CAD build for the part. Positions are in the model's coordinates, mm. A direction names the side the tool comes from. Coordinates: 2 decimals unless noted, no trailing zeros. Loops run counter-clockwise (first coordinate to the right, second up) from the corner with the lowest first, then second, coordinate; pieces in that order, holes last. Notation, with made-up numbers: (61, -19) -> (110, -19) arc R17 cw to (110, 11) -> close; hole circle Ø2 at (16, 66). An arc over 180 degrees is marked (long way). Write each question's results on one line, items separated by ' | '.
from build123d import *

# Parameters (mm, degrees)
SKETCH1_R           = 7
SKETCH1_R_2         = 1.75
BOSS_EXTRUDE1_DEPTH = 3
SKETCH2_R           = 4
SKETCH2_R_2         = 1.75
BOSS_EXTRUDE2_DEPTH = 6
FILLET1_R           = 3
SKETCH4_R           = 2.75
SKETCH4_R_2         = 1.75
BOSS_EXTRUDE3_DEPTH = 4.25


# Some blends are built 0.0001 mm under size
with BuildPart() as part:
    # Sketch1 → Boss-Extrude1 (new body)
    with BuildSketch(Plane(origin=(0, 0, 0), x_dir=(0, 0, -1), z_dir=(1, 0, 0))):
        Circle(SKETCH1_R)
        Circle(SKETCH1_R_2, mode=Mode.SUBTRACT)
    extrude(amount=BOSS_EXTRUDE1_DEPTH)

    # Sketch2 → Boss-Extrude2 (add)
    with BuildSketch(Plane(origin=(3, 0, 0), x_dir=(0, 0, -1), z_dir=(1, 0, 0))):
        Circle(SKETCH2_R)
        Circle(SKETCH2_R_2, mode=Mode.SUBTRACT)
    extrude(amount=BOSS_EXTRUDE2_DEPTH)

    # Fillet1
    fillet1_edges = [part.edges().sort_by_distance(p)[0] for p in [
        (3, 0, 4),
    ]]
    fillet(fillet1_edges, radius=FILLET1_R - 0.0001)  # a hair under: the kernel refuses the full size

    # Sketch4 → Boss-Extrude3 (add)
    with BuildSketch(Plane(origin=(9, 0, 0), x_dir=(0, 0, -1), z_dir=(1, 0, 0))):
        Circle(SKETCH4_R)
        Circle(SKETCH4_R_2, mode=Mode.SUBTRACT)
    extrude(amount=BOSS_EXTRUDE3_DEPTH)

    # Chamfer1
    # the kernel refuses this chamfer: 0.25 mm, written as the material it takes off along each edge
    with BuildSketch(Plane(origin=(9, 0, 0), x_dir=(0, 0, -1), z_dir=(0, -1, 0))) as chamfer1_piece_1:
        with BuildLine():
            Line((3.696966991, 0.053033009), (4.053033009, -0.303033009))
            Line((4.053033009, -0.303033009), (4.090533009, -0.303033009))
            ThreePointArc((4.090533009, -0.303033009), (4.0375, -0.151516504), (4.0375, 0))
            Line((4.0375, 0), (4, 0.0375))
            ThreePointArc((4, 0.0375), (3.848483496, 0.0375), (3.696966991, 0.090533009))
            Line((3.696966991, 0.090533009), (3.696966991, 0.053033009))
        make_face()
    revolve(axis=Axis((9, 0, 0), (1, 0, 0)), mode=Mode.SUBTRACT)
    with BuildSketch(Plane(origin=(0, 0, 0), x_dir=(0, 0, -1), z_dir=(0, -1, 0))) as chamfer1_piece_2:
        with BuildLine():
            Line((7.053033009, 0.303033009), (6.696966991, -0.053033009))
            Line((6.696966991, -0.053033009), (6.696966991, -0.090533009))
            ThreePointArc((6.696966991, -0.090533009), (6.848483496, -0.0375), (7, -0.0375))
            Line((7, -0.0375), (7.0375, 0))
            ThreePointArc((7.0375, 0), (7.0375, 0.151516504), (7.090533009, 0.303033009))
            Line((7.090533009, 0.303033009), (7.053033009, 0.303033009))
        make_face()
    revolve(axis=Axis((0, 0, 0), (1, 0, 0)), mode=Mode.SUBTRACT)
    with BuildSketch(Plane(origin=(13.25, 0, 0), x_dir=(0, 0, -1), z_dir=(0, -1, 0))) as chamfer1_piece_3:
        with BuildLine():
            Line((2.446966991, 0.053033009), (2.803033009, -0.303033009))
            Line((2.803033009, -0.303033009), (2.840533009, -0.303033009))
            ThreePointArc((2.840533009, -0.303033009), (2.7875, -0.151516504), (2.7875, 0))
            Line((2.7875, 0), (2.75, 0.0375))
            ThreePointArc((2.75, 0.0375), (2.598483496, 0.0375), (2.446966991, 0.090533009))
            Line((2.446966991, 0.090533009), (2.446966991, 0.053033009))
        make_face()
    revolve(axis=Axis((13.25, 0, 0), (1, 0, 0)), mode=Mode.SUBTRACT)
    with BuildSketch(Plane(origin=(3, 0, 0), x_dir=(0, 0, -1), z_dir=(0, -1, 0))) as chamfer1_piece_4:
        with BuildLine():
            Line((6.696966991, 0.053033009), (7.053033009, -0.303033009))
            Line((7.053033009, -0.303033009), (7.090533009, -0.303033009))
            ThreePointArc((7.090533009, -0.303033009), (7.0375, -0.151516504), (7.0375, 0))
            Line((7.0375, 0), (7, 0.0375))
            ThreePointArc((7, 0.0375), (6.848483496, 0.0375), (6.696966991, 0.090533009))
            Line((6.696966991, 0.090533009), (6.696966991, 0.053033009))
        make_face()
    revolve(axis=Axis((3, 0, 0), (1, 0, 0)), mode=Mode.SUBTRACT)
    with BuildSketch(Plane(origin=(0, 0, 0), x_dir=(0, 0, -1), z_dir=(0, -1, 0))) as chamfer1_piece_5:
        with BuildLine():
            Line((2.053033009, -0.053033009), (1.696966991, 0.303033009))
            Line((1.696966991, 0.303033009), (1.659466991, 0.303033009))
            ThreePointArc((1.659466991, 0.303033009), (1.7125, 0.151516504), (1.7125, 0))
            Line((1.7125, 0), (1.75, -0.0375))
            ThreePointArc((1.75, -0.0375), (1.901516504, -0.0375), (2.053033009, -0.090533009))
            Line((2.053033009, -0.090533009), (2.053033009, -0.053033009))
        make_face()
    revolve(axis=Axis((0, 0, 0), (1, 0, 0)), mode=Mode.SUBTRACT)


solid = part.part
1) Which spindle directions (+Z, -Z, +X, -X, +Y, -Y) get a long thin tool onto all of the face, cutting with end or side? Do faces 1 (the cylindrical face through (1.482, -2.681, -6.466)), 2 (the cylindrical face through (10.972, -2.685, 0.596)). Say none if no direction does.
Outcome:
face 1: +X, -X | face 2: +X
2) Drill centre lines: L1, parallel to Y at x = 7.25, z = 0; L2, parallel to Y at x = 9.75, z = 0. Where is each one in solid material? Low to high. Write a range as from..to.
Outcome:
L1: y = -4..-1.75, 1.75..4 | L2: y = -2.75..-1.75, 1.75..2.75
3) Slice it at A-A (y = 0). Write the cut outline in (x, z).
Outcome:
outline: (0, -6.75) -> (0.25, -7) -> (2.75, -7) -> (3.01, -6.74) arc R3 cw to (6, -4) -> (8.75, -4) -> (9, -3.75) -> (9, -2.75) -> (13, -2.75) -> (13.25, -2.5) -> (13.25, -1.75) -> (0.25, -1.75) -> (0, -2) -> close; (0, 2) -> (0.25, 1.75) -> (13.25, 1.75) -> (13.25, 2.5) -> (13, 2.75) -> (9, 2.75) -> (9, 3.75) -> (8.75, 4) -> (6, 4) arc R3 cw to (3.01, 6.74) -> (2.75, 7) -> (0.25, 7) -> (0, 6.75) -> close
4) Slice it at C-C (x = 1). Write the cut outline in (y, z).
Outcome:
outline: circle Ø14 at (0, 0); hole circle Ø3.5 at (0, 0)
5) Pin check, flat tips, straight feed: pin 1 (5 mm diameter, centred on x = 7.5, z = 3, fed in from -Y); pin 2 (3 mm diameter, centred on y = 0, z = 0, fed in from -X); pin 3 (2 mm diameter, centred on x = 11, z = 1, fed in from +Y); pin 4 (5 mm diameter, centred on x = 5, y = 4, fed in from +Z). Stop position of each tip, or through.
Outcome:
pin 1: stops at y = -3.97 | pin 2: passes through | pin 3: stops at y = 2.75 | pin 4: stops at z = 6.37
6) Two-plate mould, pull along Z, no slides. Class faces 3 (the flat face through (13.25, 2, -1)), 4 (the cylindrical face through (6.659, -0.67, -1.617)), 5 (the cylindrical face through (7.356, -3.905, 0.867)): pulls with the +Z half, pulls with the -Z half, needs draft (parallel to the pull), parting line crosses it, or undercut.
Outcome:
face 3: needs draft | face 4: undercut | face 5: parting line crosses it
7) Slice it at D-D (x = 4). Write the cut outline in (y, z).
Outcome:
outline: circle Ø9.53 at (0, 0); hole circle Ø3.5 at (0, 0)
